For this review, take the finished solid that the model builds, in its own axes (mm). Face numbers are marked on the shaded views. Give positions to 0.01 mm unless a question says otherwise; leave off trailing zeros. Order: outer loops, then holes, each group sorted by start corner. A loop starts at its lowest first (then second) coordinate and runs counter-clockwise, first axis right, second up. Notation, with made-up numbers: M 87.5,-4.75 L 111.5,-4.75 A13 ccw 111.5,13.25 Z; hole C 89.5,6.5 d9. An arc over 180 degrees is marked long. Use CSV: the item, a comma, the result in double quotes. Start each with the question number.
(1) Consider section B-B (z = 2.05). Write out the cut boundary in (x, y), and give its area (3 significant figures).
(2) Draft analysis for pull direction Y (two halves, no side actions). For the marked faces 1, 2, 3 and 4, state which applies: pulls with the +Y half, pulls with the -Y half, needs draft (parallel to the pull), parting line crosses it, or undercut.
(3) Consider section A-A (x = 10). Write out the cut boundary in (y, z), and give its area (3 significant figures).
(4) Consider section D-D (y = 37.5). Write out the cut boundary in (x, z), and give its area (3 significant figures).
(5) Wall thickness on L1, parallel to Y at x = 10, z = 2.25; L2, parallel to Y at x = 26, z = 4.45: over which ranges is each line inside the solid? List them lowest first. Write a range as from..to.
(6) Clearance check with a flat-ended pin moving along its axis: P1, Ø1.4, axis at y = 27.5, z = 1.5, coming from the +X side. State where the tip first meets the part, or that it passes through.
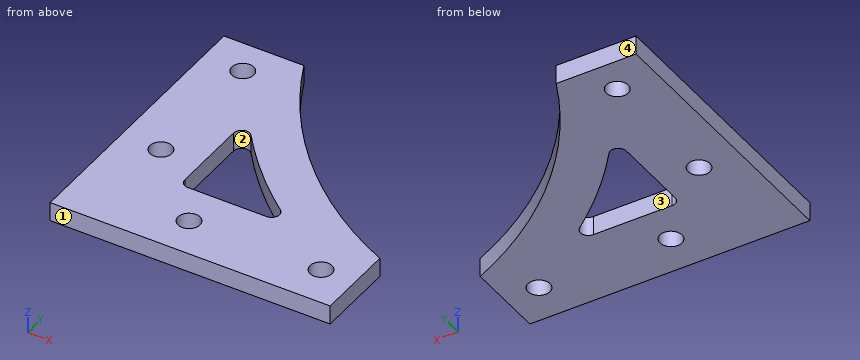
```python
from build123d import *

# Parameters (mm, degrees)
SKETCH1_R           = 2.75
BOSS_EXTRUDE1_DEPTH = 4.7625


with BuildPart() as part:
    # Sketch1 → Boss-Extrude1 (new body)
    with BuildSketch(Plane.XY):
        with BuildLine():
            Line((0, 0), (70, 0))
            Line((70, 0), (70, 20))
            ThreePointArc((70, 20), (40.433104658, 40.433104658), (20, 70))
            Line((20, 70), (0, 70))
            Line((0, 70), (0, 0))
        make_face()
        with Locations((10, 61.5)):
            Circle(SKETCH1_R, mode=Mode.SUBTRACT)
        with Locations((10, 28.5)):
            Circle(SKETCH1_R, mode=Mode.SUBTRACT)
        with Locations((28.5, 10)):
            Circle(SKETCH1_R, mode=Mode.SUBTRACT)
        with Locations((61.5, 10)):
            Circle(SKETCH1_R, mode=Mode.SUBTRACT)
        with BuildLine():
            Line((20, 41.700381418), (20, 22))
            ThreePointArc((20, 22), (20.585786438, 20.585786438), (22, 20))
            Line((22, 20), (41.700381418, 20))
            ThreePointArc((41.700381418, 20), (43.591879783, 21.350204699), (42.929468168, 23.577766067))
            ThreePointArc((42.929468168, 23.577766067), (32.654930065, 32.654930065), (23.577766067, 42.929468168))
            ThreePointArc((23.577766067, 42.929468168), (21.350204699, 43.591879783), (20, 41.700381418))
        make_face(mode=Mode.SUBTRACT)
    extrude(amount=BOSS_EXTRUDE1_DEPTH)


solid = part.part
```
Check result:
1,outline,"M 0,0 L 70,0 L 70,20 A100 cw 20,70 L 0,70 Z; hole C 10,28.5 d5.5; hole C 10,61.5 d5.5; hole M 20,22 A2 ccw 22,20 L 41.7,20 A2 ccw 42.93,23.58 A111 cw 23.58,42.93 A2 ccw 20,41.7 Z; hole C 28.5,10 d5.5; hole C 61.5,10 d5.5"
1,area,"2,920 mm^2"
2,face 1,"pulls with the -Y half"
2,face 2,"undercut"
2,face 3,"undercut"
2,face 4,"pulls with the +Y half"
3,outline,"M 0,0 L 25.75,0 L 25.75,4.76 L 0,4.76 Z; M 31.25,0 L 58.75,0 L 58.75,4.76 L 31.25,4.76 Z; M 64.25,0 L 70,0 L 70,4.76 L 64.25,4.76 Z"
3,area,"281 mm^2"
4,outline,"M 0,0 L 20,0 L 20,4.76 L 0,4.76 Z; M 28.09,0 L 43.49,0 L 43.49,4.76 L 28.09,4.76 Z"
4,area,"169 mm^2"
5,L1,"y = 0..25.75, 31.25..58.75, 64.25..70"
5,L2,"y = 0..8.85, 11.15..20, 39.93..58.7"
6,P1,"stops at x = 57.42"
